from build123d import *

# Parameters (mm, degrees)
ESQUISSE1_W        = 8.2
ESQUISSE1_H        = 7.7
BOSS_EXTRU_1_DEPTH = 4.8
ESQUISSE1_3_R      = 1.5
BOSS_EXTRU_2_DEPTH = 2.2


with BuildPart() as part:
    # Esquisse1 → Boss.-Extru.1 (new body)
    with BuildSketch(Plane(origin=(0, 0, 0), x_dir=(1, 0, 0), z_dir=(0, 1, 0))):
        Rectangle(ESQUISSE1_W, ESQUISSE1_H)
        Polygon((1.905255888, -3.3), (3.810511777, 0), (1.905255888, 3.3), (-1.905255888, 3.3), (-3.810511777, 0), (-1.905255888, -3.3), align=None, mode=Mode.SUBTRACT)
    extrude(amount=BOSS_EXTRU_1_DEPTH)

    # Esquisse1_3 → Boss.-Extru.2 (add)
    with BuildSketch(Plane(origin=(0, 0, 0), x_dir=(1, 0, 0), z_dir=(0, 1, 0))):
        Polygon((-1.905255888, -3.3), (1.905255888, -3.3), (3.810511777, 0), (1.905255888, 3.3), (-1.905255888, 3.3), (-3.810511777, 0), align=None)
        Circle(ESQUISSE1_3_R, mode=Mode.SUBTRACT)
    extrude(amount=BOSS_EXTRU_2_DEPTH)


solid = part.part
The listing builds one solid part. Answer for the finished solid, in the listing's coordinates (mm). A direction names the side the tool comes from. Coordinates: 2 decimals unless noted, no trailing zeros. Loops run counter-clockwise (first coordinate to the right, second up) from the corner with the lowest first, then second, coordinate; pieces in that order, holes last. Notation, with made-up numbers: (11, -6.75) -> (43, -6.75) arc R17 cw to (43, 0.25) -> close; hole circle Ø3 at (79.25, -40). An arc over 180 degrees is marked (long way). Answer in a Markdown table with one row per item. Add a question column.
1. A flat-ended cylindrical pin translates along its axis: P1, Ø3.5, axis at x = 1, z = -0.5, coming from the +Y side. Find the tip coordinate at first contact, or state that the pin passes through.
2. The part is cut by section A-A, the plane y = 3.8. Write down the section's boundary in (x, z).
3. Determine the mould class of faces 3 (the flat face through (0, 2.2, -2)), 4 (the flat face through (4.1, 2, 0)), 5 (the flat face through (0, 0, -2)) for opening direction X: +X half, -X half, draft (parallel to the pull), parting line (faces both ways), or undercut.
4. The part is cut by section D-D, the plane y = 1.4. Write down the section's boundary in (x, z), then the cut area to 3 significant figures.
5. The part is cut by section B-B, the plane x = 0. Write down the section's boundary in (y, z), then the cut area to 3 significant figures.
6. For faces 1 (the flat face through (2.87, 3.48, -1.63)), 2 (the flat face through (0, 2, 3.85)), determine the directions among +Z, -Z, +X, -X, +Y, -Y from which every point of the face is accessible in a straight line to the end or side of a thin tool.
7. Consider line 1 (X direction, y = 1.7, z = 0); line 2 (Z direction, x = 1.25, y = 3.45); line 3 (Y direction, x = -3, z = 0.5). Determine where each line is inside the solid, lowest interval first. Write a range as [from, to].
8. The part is cut by section C-C, the plane z = -0.5. Write down the section's boundary in (x, y), then the cut area to 3 significant figures.
Answer below:
| question | item | result |
|---|---|---|
| 1 | P1 | y = 2.2 |
| 2 | outline | (-4.1, -3.85) -> (4.1, -3.85) -> (4.1, 3.85) -> (-4.1, 3.85) -> close; hole (-3.81, 0) -> (-1.91, -3.3) -> (1.91, -3.3) -> (3.81, 0) -> (1.91, 3.3) -> (-1.91, 3.3) -> close |
| 3 | face 3 | undercut |
| 3 | face 4 | +X half |
| 3 | face 5 | draft |
| 4 | outline | (-4.1, -3.85) -> (4.1, -3.85) -> (4.1, 3.85) -> (-4.1, 3.85) -> close; hole circle Ø3 at (0, 0) |
| 4 | area | 56.1 mm2 |
| 5 | outline | (0, -3.85) -> (4.8, -3.85) -> (4.8, -3.3) -> (2.2, -3.3) -> (2.2, -1.5) -> (0, -1.5) -> close; (0, 1.5) -> (2.2, 1.5) -> (2.2, 3.3) -> (4.8, 3.3) -> (4.8, 3.85) -> (0, 3.85) -> close |
| 5 | area | 13.2 mm2 |
| 6 | face 1 | +Y |
| 6 | face 2 | +Z, +X, -X, +Y, -Y |
| 7 | line 1 | [-4.1, -1.5], [1.5, 4.1] |
| 7 | line 2 | [-3.85, -3.3], [3.3, 3.85] |
| 7 | line 3 | [0, 2.2] |
| 8 | outline | (-4.1, 0) -> (-1.41, 0) -> (-1.41, 2.2) -> (-3.52, 2.2) -> (-3.52, 4.8) -> (-4.1, 4.8) -> close; (1.41, 0) -> (4.1, 0) -> (4.1, 4.8) -> (3.52, 4.8) -> (3.52, 2.2) -> (1.41, 2.2) -> close |
| 8 | area | 14.8 mm2 |
